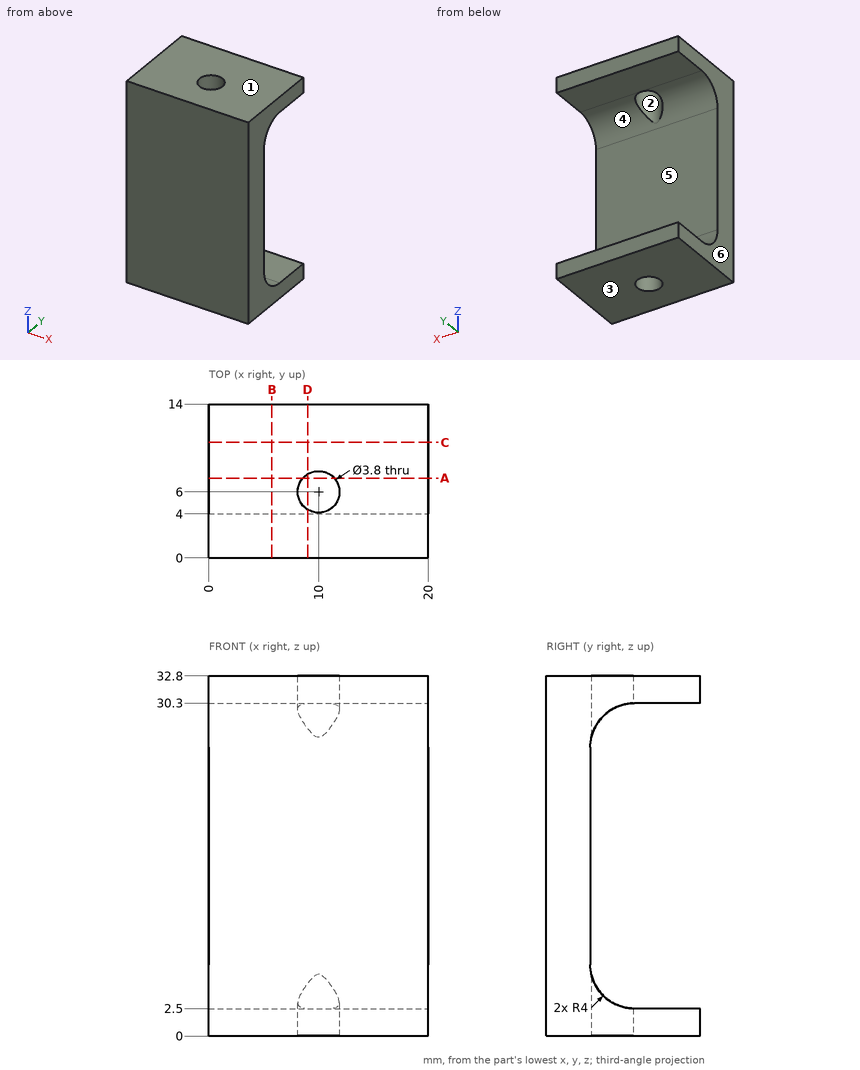
For this review, use the dimensioned drawing (mm, ordinates from the lowest corner) and the shaded views. A direction names the side the tool comes from. Round coordinates to 2 decimals unless told otherwise and drop trailing zeros. Order: outer loops, then holes, each group sorted by start corner. A loop starts at its lowest first (then second) coordinate and runs counter-clockwise, first axis right, second up.
1) For L1, parallel to Z at x = 16.5, y = 8; L2, parallel to Y at x = 10, z = 2.35; L3, parallel to X at y = 6, z = 1.6, list the stretches that pass through material, from the lowest coordinate up.
The answers:
L1: z = 0 to 2.5, 30.3 to 32.8
L2: y = 0 to 4.1, 7.9 to 14
L3: x = 0 to 8.1, 11.9 to 20
2) Consider section D-D (x = 9). State the section outline as (y, z) points, plus the area to 3 significant figures.
The answers:
outline: (0, 0) - (4.38, 0) - (4.38, 4.79) arc R4 cw to (4, 6.5) - (4, 26.3) arc R4 cw to (4.38, 28.01) - (4.38, 32.8) - (0, 32.8) - close; (7.62, 0) - (14, 0) - (14, 2.5) - (8, 2.5) arc R4 cw to (7.62, 2.52) - close; (7.62, 30.28) arc R4 cw to (8, 30.3) - (14, 30.3) - (14, 32.8) - (7.62, 32.8) - close
area: 167 mm2
3) Draft analysis for pull direction Z (two halves, no side actions). For the marked faces 1, 2, 3 and 4, state which applies: released by +Z, released by -Z, zero draft, split by the parting line, or undercut.
The answers:
face 1: released by +Z
face 2: zero draft
face 3: released by -Z
face 4: undercut
4) Clearance check with a flat-ended pin moving along its axis: pin 1 Ø8 at (x, z) = (10, 14) entering from +Y. State where the tip first meets the part, or that it passes through.
The answers:
pin 1: stops at y = 4
5) Machinability: for the marked faces 5 and 6, which of the approach directions +Z, -Z, +X, -X, +Y, -Y give a long, thin tool a straight path to every point of the face, cutting with its end or side? Answer none if there is none.
The answers:
face 5: +X, -X, +Y
face 6: +Z, -Z, -X, +Y, -Y
6) Consider section B-B (x = 5.75). State the section outline as (y, z) points, plus the area to 3 significant figures.
The answers:
outline: (0, 0) - (14, 0) - (14, 2.5) - (8, 2.5) arc R4 cw to (4, 6.5) - (4, 26.3) arc R4 cw to (8, 30.3) - (14, 30.3) - (14, 32.8) - (0, 32.8) - close
area: 188 mm2
7) Consider section A-A (y = 7.25). State the section outline as (x, z) points.
The answers:
outline: (0, 0) - (8.57, 0) - (8.57, 2.57) - (0, 2.57) - close; (0, 30.23) - (8.57, 30.23) - (8.57, 32.8) - (0, 32.8) - close; (11.43, 0) - (20, 0) - (20, 2.57) - (11.43, 2.57) - close; (11.43, 30.23) - (20, 30.23) - (20, 32.8) - (11.43, 32.8) - close
8) Consider section C-C (y = 10.5). State the section outline as (x, z) points, plus the area to 4 significant figures.
The answers:
outline: (0, 0) - (20, 0) - (20, 2.5) - (0, 2.5) - close; (0, 30.3) - (20, 30.3) - (20, 32.8) - (0, 32.8) - close
area: 100.0 mm2
